Design review of the part built by this model. Coordinates are the model's own, in mm. Coordinates: 2 decimals unless noted, no trailing zeros. Order: outer loops, then holes, each group sorted by start corner. A loop starts at its lowest first (then second) coordinate and runs counter-clockwise, first axis right, second up. Notation, with made-up numbers: (-0.75, -22.5) -> (30.25, -22.5) arc R23 ccw to (30.25, 4.5) -> close; hole circle Ø6 at (28, -19.5). An arc over 180 degrees is marked (long way). Use a Markdown table: item, result. Add a question column.
Q1. Add section B-B (y = 35). State the section outline as (x, z) points, then the cut area to 3 significant figures.
Q2. Wall thickness on probe 1 along Y at (x, z) = (-26.6, 1.65); probe 2 along X at (y, z) = (62.5, 0.9): over which ranges is each line inside the solid? List them lowest first.
Q3. Add section A-A (z = 2.5). Count the separate pieces of the cut face and the enclosed holes in it, then the cut area to 3 significant figures.
Q4. Insertion check: pin 1 (0.9 mm diameter, centred on x = -17.5, z = 1, fed in from +Y); pin 2 (1.5 mm diameter, centred on x = -17.5, z = 2, fed in from -Y); pin 3 (0.6 mm diameter, centred on y = 10.5, z = 1.5, fed in from -X). Each pin has a flat end and moves straight along its axis. Give the tip position at first contact, or say it passes through.
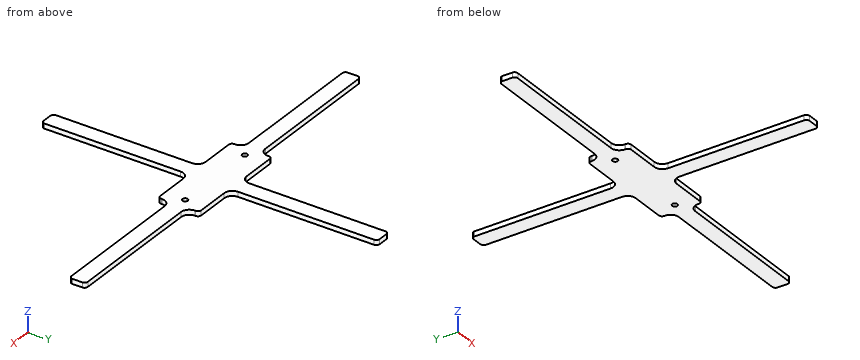
Autodesk Inventor part; units mm, degrees
ref_plane "YZ Plane" through (0, 0, 0) normal (1, 0, 0) x (0, 1, 0)
ref_plane "XZ Plane" through (0, 0, 0) normal (0, 1, 0) x (-1, 0, 0)
ref_plane "XY Plane" through (0, 0, 0) normal (0, 0, 1) x (1, 0, 0)
sketch "Sketch1" plane through (0, 0, 0) normal (0, 0, 1) x (1, 0, 0)
  line L0 (-32.5, -12.5) -> (32.5, -12.5)
  line L1 (32.5, -12.5) -> (32.5, 12.5)
  line L2 (32.5, 12.5) -> (-32.5, 12.5)
  line L3 (-32.5, 12.5) -> (-32.5, -12.5)
  line L4 (-32.5, -12.5) -> (32.5, 12.5) construction
  line L5 (32.5, -12.5) -> (-32.5, 12.5) construction
  line L6 (32.5, 5) -> (122.5, 5)
  line L7 (122.5, 5) -> (122.5, -5)
  line L8 (122.5, -5) -> (32.5, -5)
  line L9 (-5, 12.5) -> (-5, 102.5)
  line L10 (-5, 102.5) -> (5, 102.5)
  line L11 (5, 102.5) -> (5, 12.5)
  line L12 (-32.5, 5) -> (-122.5, 5)
  line L13 (-122.5, 5) -> (-122.5, -5)
  line L14 (-122.5, -5) -> (-32.5, -5)
  line L15 (-5, -12.5) -> (-5, -102.5)
  line L16 (-5, -102.5) -> (5, -102.5)
  line L17 (5, -102.5) -> (5, -12.5)
  circle A0 centre (-26.6, 0) radius 1.6
  circle A1 centre (26.6, 0) radius 1.6
  line L18 (0, 0) -> (0, 12.5) construction
  line L19 (-26.6, 0) -> (26.6, 0) construction
  dimension "d0" = 90
  dimension "d1" = 53.2
  dimension "d2" = 10
  dimension "d3" = 3.2
  dimension "d4" = 65
  dimension "d5" = 25
  dimension "d6" = 90
extrude "Extrusion1" add sketch "Sketch1" along normal blind 3
fillet "Fillet1" radius 2 12 edges at (32.5, 12.5, 1.5) (5, 102.5, 1.5) (-5, 102.5, 1.5) (-122.5, 5, 1.5) (-122.5, -5, 1.5) (-32.5, 12.5, 1.5) (-32.5, -12.5, 1.5) (-5, -102.5, 1.5) (5, -102.5, 1.5) (32.5, -12.5, 1.5) (122.5, -5, 1.5) (122.5, 5, 1.5)
fillet "Fillet1" radius 5 8 edges at (5, -12.5, 1.5) (-5, -12.5, 1.5) (32.5, -5, 1.5) (32.5, 5, 1.5) (5, 12.5, 1.5) (-5, 12.5, 1.5) (-32.5, -5, 1.5) (-32.5, 5, 1.5)
properties part number "spin_light_tester"
Established:
| question | item | result |
|---|---|---|
| 1 | outline | (-5, 0) -> (5, 0) -> (5, 3) -> (-5, 3) -> close |
| 1 | area | 30.0 mm^2 |
| 2 | probe 1 | -12.5 to -1.6, 1.6 to 12.5 |
| 2 | probe 2 | -5 to 5 |
| 3 | separate pieces | 1 |
| 3 | enclosed holes | 2 |
| 3 | area | 5,240 mm^2 |
| 4 | pin 1 | y = 12.5 |
| 4 | pin 2 | y = -12.5 |
| 4 | pin 3 | x = -32.5 |
